CAD build for the part. Positions are in the model's coordinates, mm. A direction names the side the tool comes from. Give positions to 0.01 mm unless a question says otherwise; leave off trailing zeros. Order: outer loops, then holes, each group sorted by start corner. A loop starts at its lowest first (then second) coordinate and runs counter-clockwise, first axis right, second up.
from build123d import *

# Parameters (mm, degrees)
F0_R     = 12
F1_DEPTH = 40
F0_R_2   = 45.49902
F2_DEPTH = 5
F3_DEPTH = 226
F0_R_3   = 5.5
F4_DEPTH = 22


with BuildPart() as f1:
    # F0 (on Right) → F1 (new body)
    with BuildSketch(Plane.YZ):
        Circle(F0_R)
    extrude(amount=-F1_DEPTH)

    # F0 (on Right) → F2 (join)
    with BuildSketch(Plane.YZ):
        Circle(F0_R_2)
        Circle(F0_R, mode=Mode.SUBTRACT)
    extrude(amount=-F2_DEPTH)

    # F0 (on Right) → F3 (join)
    with BuildSketch(Plane.YZ):
        with BuildLine():
            Line((-39.6, -65), (39.6, -65))
            Line((39.6, -65), (39.6, -52.3))
            ThreePointArc((39.6, -52.3), (43.3197438789, -43.3197438789), (52.3, -39.6))
            Line((52.3, -39.6), (65, -39.6))
            Line((65, -39.6), (65, 39.6))
            Line((65, 39.6), (52.3, 39.6))
            ThreePointArc((52.3, 39.6), (43.3197438789, 43.3197438789), (39.6, 52.3))
            Line((39.6, 52.3), (39.6, 65))
            Line((39.6, 65), (-39.6, 65))
            Line((-39.6, 65), (-39.6, 52.3))
            ThreePointArc((-39.6, 52.3), (-43.3197438789, 43.3197438789), (-52.3, 39.6))
            Line((-52.3, 39.6), (-65, 39.6))
            Line((-65, 39.6), (-65, -39.6))
            Line((-65, -39.6), (-52.3, -39.6))
            ThreePointArc((-52.3, -39.6), (-43.3197438789, -43.3197438789), (-39.6, -52.3))
            Line((-39.6, -52.3), (-39.6, -65))
        make_face()
        Circle(F0_R_2, mode=Mode.SUBTRACT)
        Circle(F0_R_2)
        Circle(F0_R, mode=Mode.SUBTRACT)
    extrude(amount=F3_DEPTH)

    # F0 (on Right) → F4 (join)
    with BuildSketch(Plane.YZ):
        with BuildLine():
            Line((-65, 52.3), (-65, 39.6))
            Line((-65, 39.6), (-52.3, 39.6))
            ThreePointArc((-52.3, 39.6), (-43.3197438789, 43.3197438789), (-39.6, 52.3))
            Line((-39.6, 52.3), (-39.6, 65))
            Line((-39.6, 65), (-52.3, 65))
            ThreePointArc((-52.3, 65), (-61.2802561211, 61.2802561211), (-65, 52.3))
        make_face()
        with Locations((-51.99888, 51.99888)):
            Circle(F0_R_3, mode=Mode.SUBTRACT)
        with BuildLine():
            Line((52.3, 39.6), (65, 39.6))
            Line((65, 39.6), (65, 52.3))
            ThreePointArc((65, 52.3), (61.2802561211, 61.2802561211), (52.3, 65))
            Line((52.3, 65), (39.6, 65))
            Line((39.6, 65), (39.6, 52.3))
            ThreePointArc((39.6, 52.3), (43.3197438789, 43.3197438789), (52.3, 39.6))
        make_face()
        with Locations((52.3, 52.3)):
            Circle(F0_R_3, mode=Mode.SUBTRACT)
        with BuildLine():
            Line((39.6, -65), (52.3, -65))
            ThreePointArc((52.3, -65), (61.2802561211, -61.2802561211), (65, -52.3))
            Line((65, -52.3), (65, -39.6))
            Line((65, -39.6), (52.3, -39.6))
            ThreePointArc((52.3, -39.6), (43.3197438789, -43.3197438789), (39.6, -52.3))
            Line((39.6, -52.3), (39.6, -65))
        make_face()
        with Locations((52.3, -52.3)):
            Circle(F0_R_3, mode=Mode.SUBTRACT)
        with BuildLine():
            Line((-52.3, -65), (-39.6, -65))
            Line((-39.6, -65), (-39.6, -52.3))
            ThreePointArc((-39.6, -52.3), (-43.3197438789, -43.3197438789), (-52.3, -39.6))
            Line((-52.3, -39.6), (-65, -39.6))
            Line((-65, -39.6), (-65, -52.3))
            ThreePointArc((-65, -52.3), (-61.2802561211, -61.2802561211), (-52.3, -65))
        make_face()
        with Locations((-51.99888, -51.99888)):
            Circle(F0_R_3, mode=Mode.SUBTRACT)
    extrude(amount=F4_DEPTH)


solid = f1.part
1. Mould opens along Y. For faces 6 (the cylindrical face through (10.85, -53.19, -57.37)), 7 (the flat face through (123, -59, 39.6)), 8 (the flat face through (111, -65, 1)) say: released by +Y, released by -Y, zero draft, split by the parting line, or undercut.
2. Saw through at B-B on y = 0. Give the cut face in (x, z).
3. Wall check: line 1 (Y direction, x = 16, z = 52); line 2 (Z direction, x = 9, y = 52); line 3 (Y direction, x = 11, z = -54.5). Give the ranges that are in metal, low to high.
4. Saw through at A-A on x = 53. Give the cut face in (y, z).
5. Saw through at D-D on x = -20.5. Give the cut face in (y, z), plus the area to 3 significant figures.
6. Pin check, flat tips, straight feed: P1, Ø1.5, axis at y = 49, z = 13, coming from the -X side; P2, Ø7, axis at y = 1, z = 6, coming from the +X side; P3, Ø6.5, axis at x = 133, y = -58.5, coming from the -Z side. Stop position of each tip, or through.
7. 3-axis set-ups, long thin cutter, end or side, ignore diameter. For faces 1 (the flat face through (123, 59, -39.6)), 2 (the cylindrical face through (111.42, -11.99, 0.53)), 3 (the flat face through (111, 1, 65)), 4 (the cylindrical face through (-22.26, -11.99, 0.53)), 5 (the flat face through (123, -59, -39.6)): which of +Z, -Z, +X, -X, +Y, -Y reach the whole face in a straight line?
Reported:
1. face 6: undercut
1. face 7: zero draft
1. face 8: released by -Y
2. outline: (-40, -12) - (-5, -12) - (-5, -45.5) - (0, -45.5) - (0, -65) - (226, -65) - (226, -12) - (0, -12) - (0, 12) - (226, 12) - (226, 65) - (0, 65) - (0, 45.5) - (-5, 45.5) - (-5, 12) - (-40, 12) - close
3. line 1: y = -65 to -57.5, -46.5 to 46.81, 57.79 to 65
3. line 2: z = -65 to -57.79, -46.81 to 46.81, 57.79 to 65
3. line 3: y = -64.81 to -56.9, -47.1 to 47.26, 57.34 to 64.81
4. outline: (-65, -39.6) - (-52.3, -39.6) arc R12.7 cw to (-39.6, -52.3) - (-39.6, -65) - (39.6, -65) - (39.6, -52.3) arc R12.7 cw to (52.3, -39.6) - (65, -39.6) - (65, 39.6) - (52.3, 39.6) arc R12.7 cw to (39.6, 52.3) - (39.6, 65) - (-39.6, 65) - (-39.6, 52.3) arc R12.7 cw to (-52.3, 39.6) - (-65, 39.6) - close; hole circle Ø24 at (0, 0)
5. outline: circle Ø24 at (0, 0)
5. area: 452 mm2
6. P1: stops at x = 0
6. P2: stops at x = 0
6. P3: stops at z = -39.6
7. face 1: -Z, +X, +Y
7. face 2: +X
7. face 3: +Z, +X, -X, +Y, -Y
7. face 4: -X
7. face 5: -Z, +X, -Y
